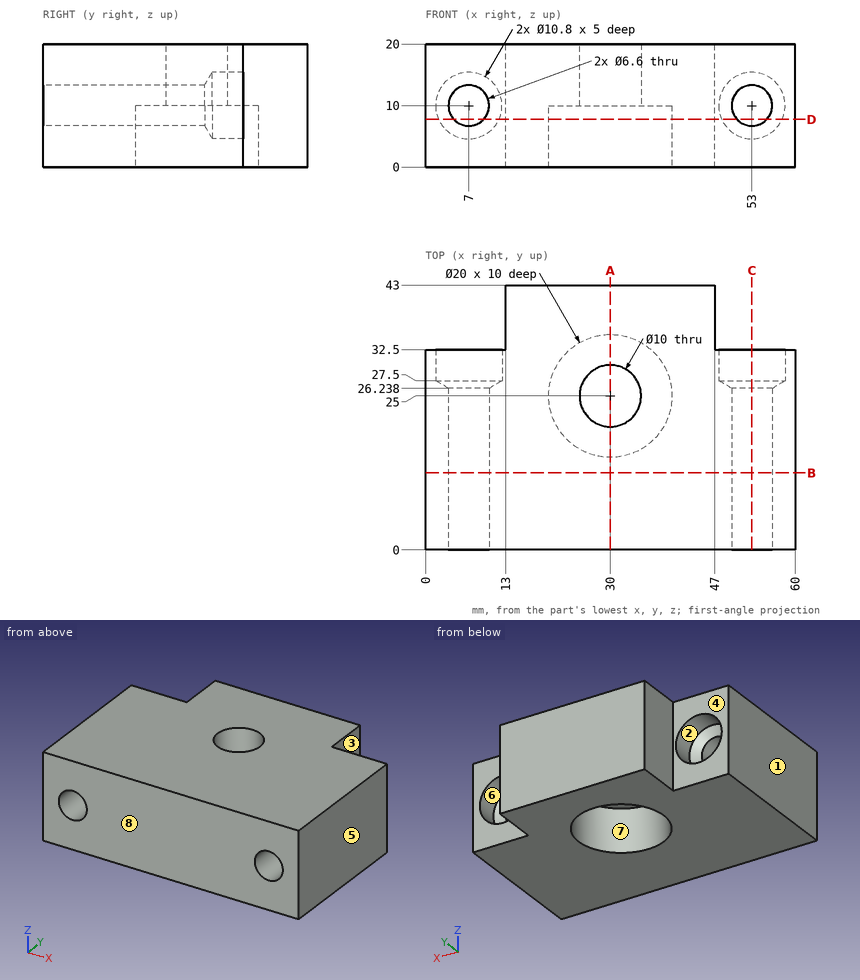
For this review, use the dimensioned drawing (mm, ordinates from the lowest corner) and the shaded views. A direction names the side the tool comes from. Round coordinates to 2 decimals unless told otherwise and drop trailing zeros. Order: outer loops, then holes, each group sorted by start corner. A loop starts at its lowest first (then second) coordinate and runs counter-clockwise, first axis right, second up. Notation, with made-up numbers: (41, -28.75) -> (46, -28.75) arc R13 ccw to (46, -21.75) -> close; hole circle Ø10 at (-33.5, -35.75). An arc over 180 degrees is marked (long way). Write item = value, one per line. Start each with the question number.
Item 1: For line 1 along X through (y, z) = (9, 10); line 2 along Z through (x, y) = (53, 6); line 3 along X through (y, z) = (17.5, 12.5) (1 decimal), list the stretches that pass through material, from the lowest coordinate up.
Item 2: For the marked faces 1, 2, 3, 4 and 5, list the 3-axis set-ups (+Z, -Z, +X, -X, +Y, -Y) from which the entire face can be reached by the end or side of a thin tool; tool diameter is ignored.
Item 3: Consider section A-A on x = 30. Write out the cut boundary in (y, z).
Item 4: Consider section C-C on x = 53. Write out the cut boundary in (y, z), plus the area to 3 significant figures.
Item 5: Mouldability with a two-part tool opening along Y and no side actions: class the marked faces 6, 7 and 8 as released by +Y, released by -Y, zero draft, split by the parting line, or undercut.
Item 6: Clearance check with flat-ended pins moving along their axes: pin 1 Ø16 at (x, y) = (30, 25) entering from -Z; pin 2 Ø3 at (y, z) = (39.5, 9.5) entering from +X; pin 3 Ø8 at (x, y) = (30, 25) entering from -Z; pin 4 Ø10.5 at (x, z) = (53, 13) entering from +Y. State where each tip first meets the part, or that it passes through.
Item 7: Consider section D-D on z = 7.75. Count the separate pieces of the cut face and the enclosed holes in it, plus the area to 3 significant figures.
Item 8: Consider section B-B on y = 12.5. Write out the cut boundary in (x, z), plus the area to 3 significant figures.
Conclusion:
q1.line_1 = 0 to 3.7, 10.3 to 49.7, 56.3 to 60
q1.line_2 = 0 to 6.7, 13.3 to 20
q1.line_3 = 0 to 4.8, 9.2 to 50.8, 55.2 to 60
q2.face_1 = +Z, -Z, -X, +Y, -Y
q2.face_2 = +Y
q2.face_3 = +Z, -Z, +X, +Y
q2.face_4 = +Z, -Z, -X, +Y
q2.face_5 = +Z, -Z, +X, +Y, -Y
q3.outline = (0, 0) -> (15, 0) -> (15, 10) -> (20, 10) -> (20, 20) -> (0, 20) -> close; (30, 10) -> (35, 10) -> (35, 0) -> (43, 0) -> (43, 20) -> (30, 20) -> close
q4.outline = (0, 0) -> (32.5, 0) -> (32.5, 4.6) -> (27.5, 4.6) -> (26.24, 6.7) -> (0, 6.7) -> close; (0, 13.3) -> (26.24, 13.3) -> (27.5, 15.4) -> (32.5, 15.4) -> (32.5, 20) -> (0, 20) -> close
q4.area = 412 mm2
q5.face_6 = zero draft
q5.face_7 = undercut
q5.face_8 = released by -Y
q6.pin_1 = 10
q6.pin_2 = 47
q6.pin_3 = through
q6.pin_4 = 32.5
q7.separate_pieces = 3
q7.enclosed_holes = 1
q7.area = 1,620 mm2
q8.outline = (0, 0) -> (60, 0) -> (60, 20) -> (0, 20) -> close; hole circle Ø6.6 at (7, 10); hole circle Ø6.6 at (53, 10)
q8.area = 1,130 mm2
